The figure shows three views and two pictorial views of one solid part (mm, origin at its lowest corner). Answer the questions. A direction names the side the tool comes from. Coordinates: 2 decimals unless noted, no trailing zeros. Loops run counter-clockwise (first coordinate to the right, second up) from the corner with the lowest first, then second, coordinate; pieces in that order, holes last. Notation, with made-up numbers: (-1, 54.5) - (20, 54.5) arc R11 ccw to (20, 75.5) - close; hole circle Ø9 at (27, 68). An arc over 180 degrees is marked (long way). Write each question's results on one line, items separated by ' | '. Start each with the question number.
Item 1: For a pull along X with two mould halves and no side action, classify the marked faces 1, 2 and 3 as +X half, -X half, draft (parallel to the pull), parting line (faces both ways), or undercut.
Item 2: Consider probe 1 along X at (y, z) = (4.15, 5); probe 2 along X at (y, z) = (0.7, 4.75); probe 3 along Y at (x, z) = (23.5, 6.5). Determine where each line is inside the solid, lowest interval first. Write a range as [from, to].
Item 3: Section D-D, the plane x = 6.5 is taken. Write down the section's boundary in (y, z).
Item 4: Section B-B, the plane y = 3.7 is taken. Write down the section's boundary in (x, z).
Item 5: Each of these flat-tipped pins is pushed along its axis until it touches: pin 1 Ø1 at (y, z) = (3.5, 7) entering from +X; pin 2 Ø3 at (y, z) = (3, 1.5) entering from -X; pin 3 Ø2.5 at (x, y) = (22, 0.5) entering from +Z. Where does it stop, or does it pass through?
Item 6: Section A-A, the plane z = 6 is taken. Write down the section's boundary in (x, y).
Item 7: A tool of negligible diameter and unlimited length cuts with its end or side. For the marked faces 4, 5 and 6, from which of +Z, -Z, +X, -X, +Y, -Y can it reach the whole face along a straight path? Write none if from no direction.
Item 8: Section C-C, the plane y = 0.8 is taken. Write down the section's boundary in (x, z).
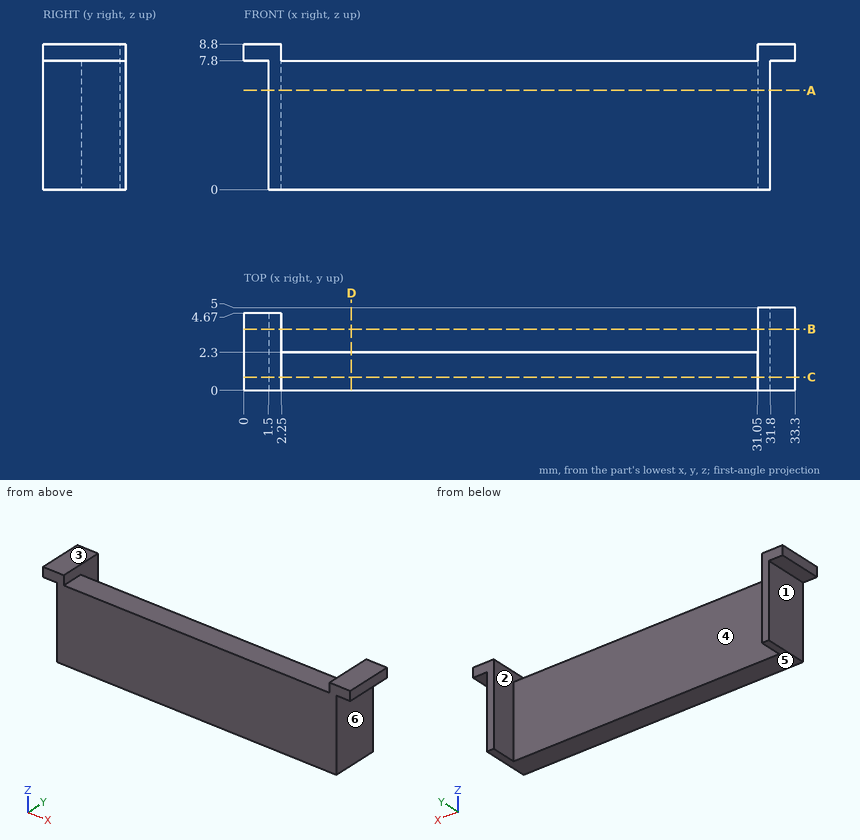
Answer key:
1) face 1: -X half | face 2: undercut | face 3: draft
2) probe 1: x = [1.5, 2.25], [31.05, 31.8] | probe 2: x = [1.5, 31.8] | probe 3: y = [0, 2.3]
3) outline: (0, 0) - (2.3, 0) - (2.3, 7.8) - (0, 7.8) - close
4) outline: (0, 7.8) - (1.5, 7.8) - (1.5, 0) - (2.25, 0) - (2.25, 8.8) - (0, 8.8) - close; (31.05, 0) - (31.8, 0) - (31.8, 7.8) - (33.3, 7.8) - (33.3, 8.8) - (31.05, 8.8) - close
5) pin 1: stops at x = 31.8 | pin 2: stops at x = 1.5 | pin 3: stops at z = 7.8
6) outline: (1.5, 0) - (31.8, 0) - (31.8, 5) - (31.05, 5) - (31.05, 2.3) - (2.25, 2.3) - (2.25, 4.67) - (1.5, 4.67) - close
7) face 4: +Z, -Z, +Y | face 5: -Z, +X, -X, +Y, -Y | face 6: -Z, +X, +Y, -Y
8) outline: (0, 7.8) - (1.5, 7.8) - (1.5, 0) - (31.8, 0) - (31.8, 7.8) - (33.3, 7.8) - (33.3, 8.8) - (31.05, 8.8) - (31.05, 7.8) - (2.25, 7.8) - (2.25, 8.8) - (0, 8.8) - close
